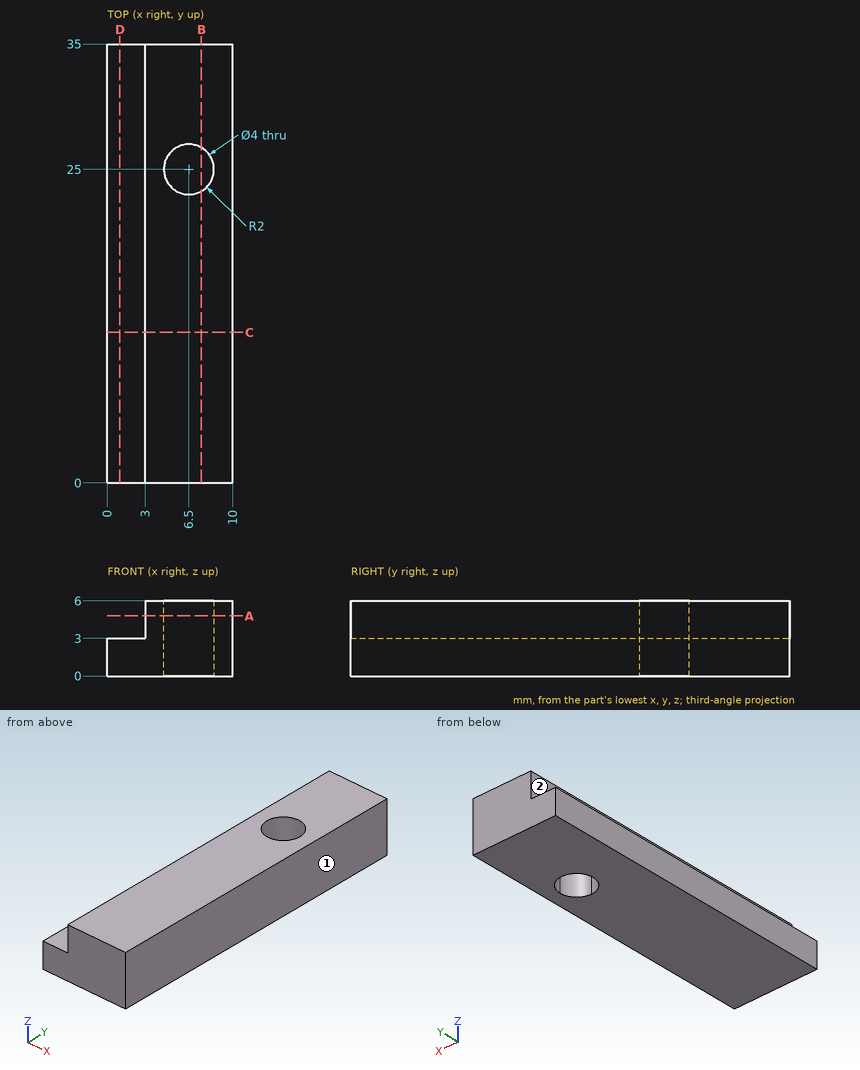
Can you work these out from the drawing? Everything is in mm from the part's minimum corner. A direction names the side the tool comes from. Coordinates: 2 decimals unless noted, no trailing zeros. Write each loop counter-clockwise with the first axis right and the second up, starting at its lowest first coordinate (ties: lowest second). Pieces come first, ordered by that corner, then holes. Notation, with made-up numbers: (-28, 12.25) -> (-3, 12.25) arc R19 ccw to (-3, 35.25) -> close; hole circle Ø8 at (48, 27). An arc over 180 degrees is marked (long way). Write each question's results on one line, items separated by ' | '. Start each with the question number.
Q1. Imagine slicing it at A-A (z = 4.8). Write out the boundary of the cut face in (x, y), then the cut area to 3 significant figures.
Q2. Imagine slicing it at C-C (y = 12). Write out the boundary of the cut face in (x, z), then the cut area to 3 significant figures.
Q3. Imagine slicing it at B-B (x = 7.5). Write out the boundary of the cut face in (y, z).
Q4. On a 3-axis mill with a long thin cutter (end or side, diameter ignored), from which of +Z, -Z, +X, -X, +Y, -Y can I reach the whole of each face in a straight line? I mean the marked faces 1 and 2. Say none if no direction works.
Q5. Imagine slicing it at D-D (x = 1). Write out the boundary of the cut face in (y, z).
Q6. I'm going to push flat-ended pins straight in: pin 1 (1.5 mm diameter, centred on x = 1.5, y = 17, fed in from +Z); pin 2 (3.5 mm diameter, centred on x = 6.5, y = 25, fed in from +Z); pin 3 (1.5 mm diameter, centred on y = 25, z = 4, fed in from -X). Where does each tip first touch, or does it pass through?
Q7. If I drill on probe 1 along X at (y, z) = (25, 1.65); probe 2 along Y at (x, z) = (6.5, 2.9); probe 3 along X at (y, z) = (25, 3.9), over which ranges is the centre line in solid material (lowest first)?
Taken from the geometry:
1) outline: (3, 0) -> (10, 0) -> (10, 35) -> (3, 35) -> close; hole (6.5, 23) arc R2 ccw to (8.5, 25) arc R2 ccw (long way) to start | area: 232 mm^2
2) outline: (0, 0) -> (10, 0) -> (10, 6) -> (3, 6) -> (3, 3) -> (0, 3) -> close | area: 51.0 mm^2
3) outline: (0, 0) -> (23.27, 0) -> (23.27, 6) -> (0, 6) -> close; (26.73, 0) -> (35, 0) -> (35, 6) -> (26.73, 6) -> close
4) face 1: +Z, -Z, +X, +Y, -Y | face 2: +Z, -X, +Y, -Y
5) outline: (0, 0) -> (35, 0) -> (35, 3) -> (0, 3) -> close
6) pin 1: stops at z = 3 | pin 2: passes through | pin 3: stops at x = 3
7) probe 1: x = 0 to 4.5, 8.5 to 10 | probe 2: y = 0 to 23, 27 to 35 | probe 3: x = 3 to 4.5, 8.5 to 10
